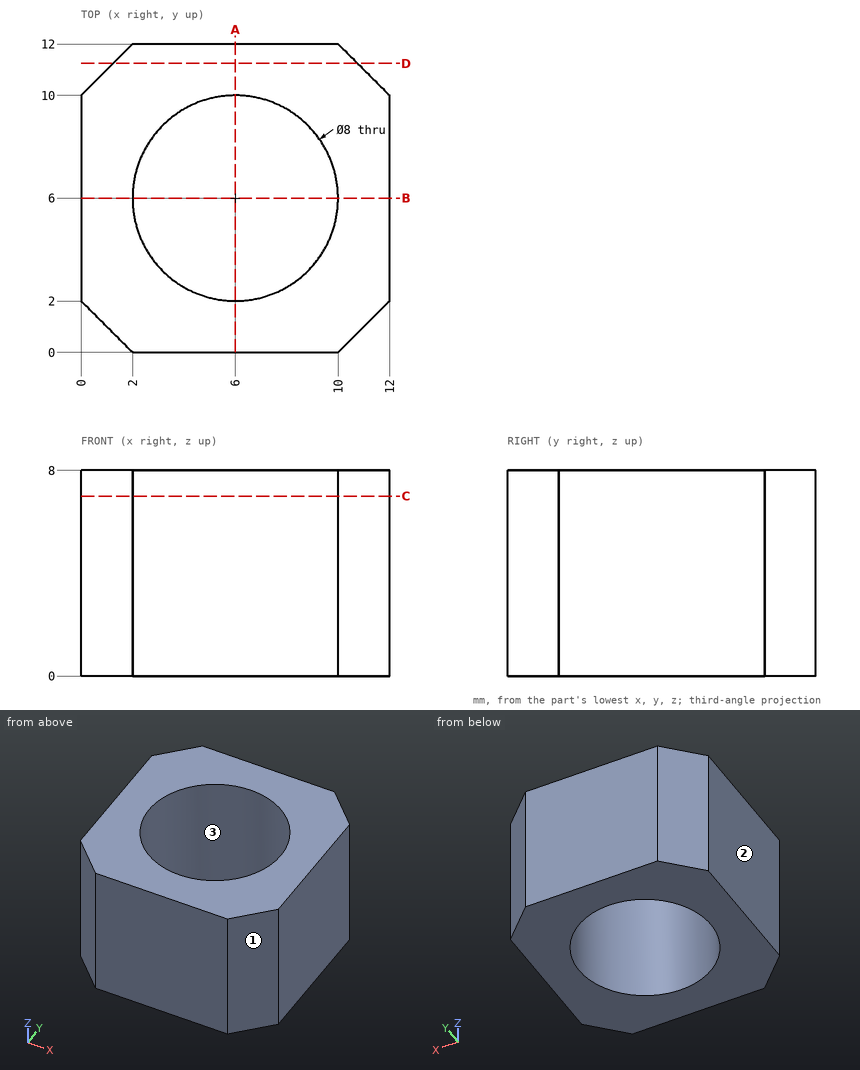
For this review, use the dimensioned drawing (mm, ordinates from the lowest corner) and the shaded views. Coordinates: 2 decimals unless noted, no trailing zeros. Order: outer loops, then holes, each group sorted by start corner. A loop starts at its lowest first (then second) coordinate and runs counter-clockwise, first axis right, second up. Notation, with made-up numbers: (65, 14) -> (75, 14) arc R31 ccw to (75, 45) -> close; hole circle Ø4 at (65, -34). An arc over 180 degrees is marked (long way). One line per item, written item: value. Start each with the question number.
Q1. Take a section at D-D, the plane y = 11.25. State the section outline as (x, z) points, then the cut area to 3 significant figures.
Q2. Take a section at C-C, the plane z = 7. State the section outline as (x, y) points.
Q3. Insertion check: pin 1 Ø4 at (x, z) = (2, 7) entering from -Y. The pin has a flat end and moves straight along its axis. Give the tip position at first contact, or say it passes through.
Q4. Mouldability with a two-part tool opening along X and no side actions: class the marked faces 1, 2 and 3 as pulls with the +X half, pulls with the -X half, needs draft (parallel to the pull), parting line crosses it, or undercut.
Q5. Take a section at A-A, the plane x = 6. State the section outline as (y, z) points, then the cut area to 3 significant figures.
Q6. For probe 1 along Y at (x, z) = (6, 4.75); probe 2 along Y at (x, z) = (3, 1); probe 3 along X at (y, z) = (5, 2.5), list the stretches that pass through material, from the lowest coordinate up.
Values follow:
1. outline: (1.25, 0) -> (10.75, 0) -> (10.75, 8) -> (1.25, 8) -> close
1. area: 76.0 mm2
2. outline: (0, 2) -> (2, 0) -> (10, 0) -> (12, 2) -> (12, 10) -> (10, 12) -> (2, 12) -> (0, 10) -> close; hole circle Ø8 at (6, 6)
3. pin 1: stops at y = 0
4. face 1: pulls with the +X half
4. face 2: pulls with the -X half
4. face 3: undercut
5. outline: (0, 0) -> (2, 0) -> (2, 8) -> (0, 8) -> close; (10, 0) -> (12, 0) -> (12, 8) -> (10, 8) -> close
5. area: 32.0 mm2
6. probe 1: y = 0 to 2, 10 to 12
6. probe 2: y = 0 to 3.35, 8.65 to 12
6. probe 3: x = 0 to 2.13, 9.87 to 12
